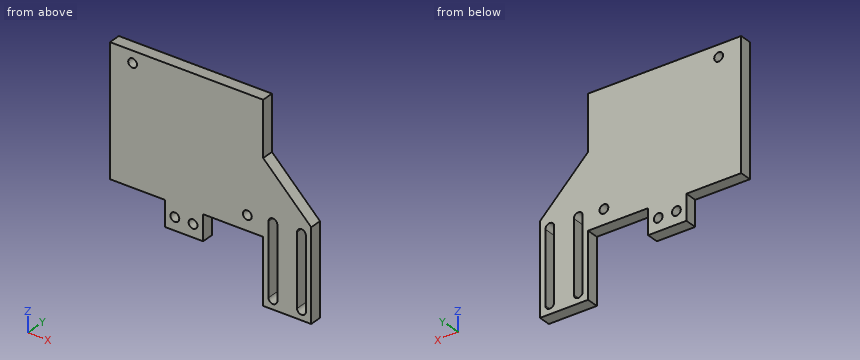
from build123d import *

# Parameters (mm, degrees)
F0_R     = 1.7
F1_DEPTH = 4.6


with BuildPart() as f1:
    # F0 (on Front) → F1 (new body)
    with BuildSketch(Plane.XZ):
        Polygon((0, 49.6), (-59, 49.6), (-59, 0), (-37.9, 0), (-37.9, -9.8), (-23.15, -9.8), (-23.15, 0), (0, 0), (0, -25), (18.5, -25), (18.5, 10), (0, 28.5), align=None)
        with Locations((-34.025, -4.9)):
            Circle(F0_R, mode=Mode.SUBTRACT)
        with Locations((-27.025, -4.9)):
            Circle(F0_R, mode=Mode.SUBTRACT)
        with BuildLine():
            Line((2.05, -21.3), (2.05, 6.3))
            ThreePointArc((2.05, 6.3), (3.75, 8), (5.45, 6.3))
            Line((5.45, 6.3), (5.45, -21.3))
            ThreePointArc((5.45, -21.3), (3.75, -23), (2.05, -21.3))
        make_face(mode=Mode.SUBTRACT)
        with BuildLine():
            Line((16.45, 6.3), (16.45, -21.3))
            ThreePointArc((16.45, -21.3), (14.75, -23), (13.05, -21.3))
            Line((13.05, -21.3), (13.05, 6.3))
            ThreePointArc((13.05, 6.3), (14.75, 8), (16.45, 6.3))
        make_face(mode=Mode.SUBTRACT)
        with Locations((-6.1, 5.7)):
            Circle(F0_R, mode=Mode.SUBTRACT)
        with Locations((-50.3, 45.1)):
            Circle(F0_R, mode=Mode.SUBTRACT)
    extrude(amount=F1_DEPTH)


solid = f1.part
Design review of the part built by this model. Coordinates are the model's own, in mm. Coordinates: 2 decimals unless noted, no trailing zeros. Write each loop counter-clockwise with the first axis right and the second up, starting at its lowest first coordinate (ties: lowest second). Pieces come first, ordered by that corner, then holes. Notation, with made-up numbers: (87.25, -26.75) - (114.25, -26.75) arc R26 cw to (114.25, 9.25) - close; hole circle Ø9 at (-35.5, -14.5). An arc over 180 degrees is marked (long way). One line per item, written item: value.
1) Add section A-A (x = -6.1). State the section outline as (y, z) points.
Answer sheet:
outline: (-4.6, 0) - (0, 0) - (0, 4) - (-4.6, 4) - close; (-4.6, 7.4) - (0, 7.4) - (0, 49.6) - (-4.6, 49.6) - close
2) Add section D-D (y = -3.8). State the section outline as (x, z) points (3 decimals).
Answer sheet:
outline: (-59, 0) - (-37.9, 0) - (-37.9, -9.8) - (-23.15, -9.8) - (-23.15, 0) - (0, 0) - (0, -25) - (18.5, -25) - (18.5, 10) - (0, 28.5) - (0, 49.6) - (-59, 49.6) - close; hole circle Ø3.4 at (-50.3, 45.1); hole circle Ø3.4 at (-34.025, -4.9); hole circle Ø3.4 at (-27.025, -4.9); hole circle Ø3.4 at (-6.1, 5.7); hole (2.05, -21.3) arc R1.7 ccw to (5.45, -21.3) - (5.45, 6.3) arc R1.7 ccw to (2.05, 6.3) - close; hole (13.05, -21.3) arc R1.7 ccw to (16.45, -21.3) - (16.45, 6.3) arc R1.7 ccw to (13.05, 6.3) - close
3) To check wall thickness, follow probe 1 along X at (y, z) = (-3.85, -9); probe 2 along Z at (x, y) = (-6, -0.85). State the ranges of each line that lie inside material, in increasing order.
Answer sheet:
probe 1: x = -37.9 to -23.15, 0 to 2.05, 5.45 to 13.05, 16.45 to 18.5
probe 2: z = 0 to 4, 7.4 to 49.6
4) Add section B-B (z = -4.9). State the section outline as (x, y) points (3 decimals).
Answer sheet:
outline: (-37.9, -4.6) - (-35.725, -4.6) - (-35.725, 0) - (-37.9, 0) - close; (-32.325, -4.6) - (-28.725, -4.6) - (-28.725, 0) - (-32.325, 0) - close; (-25.325, -4.6) - (-23.15, -4.6) - (-23.15, 0) - (-25.325, 0) - close; (0, -4.6) - (2.05, -4.6) - (2.05, 0) - (0, 0) - close; (5.45, -4.6) - (13.05, -4.6) - (13.05, 0) - (5.45, 0) - close; (16.45, -4.6) - (18.5, -4.6) - (18.5, 0) - (16.45, 0) - close
5) Add section C-C (z = -16). State the section outline as (x, y) points, plus the area to 3 significant figures.
Answer sheet:
outline: (0, -4.6) - (2.05, -4.6) - (2.05, 0) - (0, 0) - close; (5.45, -4.6) - (13.05, -4.6) - (13.05, 0) - (5.45, 0) - close; (16.45, -4.6) - (18.5, -4.6) - (18.5, 0) - (16.45, 0) - close
area: 53.8 mm2
6) Insertion check: pin 1 (2.5 mm diameter, centred on y = -1.5, z = -16.5, fed in from -X); pin 2 (2.5 mm diameter, centred on y = -3, z = -6.5, fed in from -X); pin 3 (2 mm diameter, centred on x = -27.025, z = -4.9, fed in from +Y). Each pin has a flat end and moves straight along its axis. Give the tip position at first contact, or say it passes through.
Answer sheet:
pin 1: stops at x = 0
pin 2: stops at x = -37.9
pin 3: passes through
